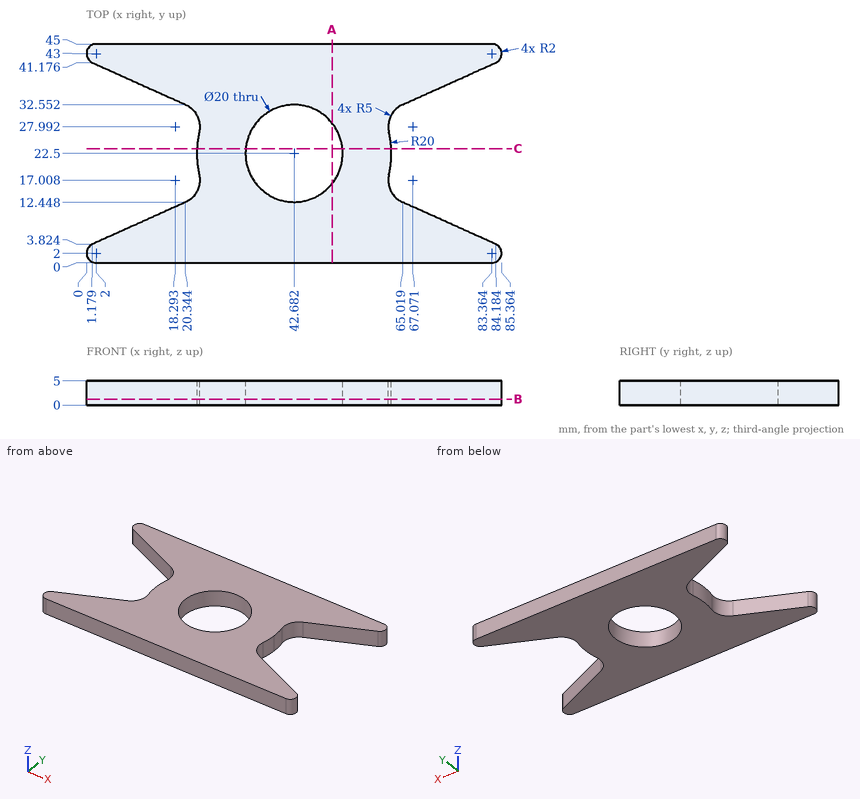
Design review of the part shown in the three views and the two pictorial views. Dimensions are in mm from the part's minimum x, y and z. Round coordinates to 2 decimals unless told otherwise and drop trailing zeros. Loops run counter-clockwise (first coordinate to the right, second up) from the corner with the lowest first, then second, coordinate; pieces in that order, holes last. Notation, with made-up numbers: (-2.75, 40) - (3.25, 40) arc R5 ccw to (3.25, 46) - close; hole circle Ø10 at (62.5, 20.5). An arc over 180 degrees is marked (long way). Write each question's results on one line, items separated by ' | '. Start each with the question number.
Q1. Insertion check: P1, Ø1.5, axis at y = 28, z = 1.5, coming from the -X side (1 decimal); P2, Ø1.5, axis at y = 27, z = 3, coming from the +X side. Each pin has a flat end and moves straight along its axis. Give the tip position at first contact, or say it passes through.
Q2. Wall thickness on line 1 along Y through (x, z) = (71, 4.55); line 2 along Y through (x, z) = (12.5, 2.15); line 3 along X through (y, z) = (29, 1.4) (1 decimal): over which ranges is each line inside the solid? List them lowest first. Write a range as [from, to].
Q3. Take a section at A-A on x = 50.5. Give the boundary of the cut face in (y, z) (1 decimal), plus the area to 3 significant figures.
Q4. Take a section at C-C on y = 23.5. Give the boundary of the cut face in (x, z).
Q5. Take a section at B-B on z = 1.25. Give the boundary of the cut face in (x, y) (1 decimal), plus the area to 3 significant figures.
Data:
1) P1: stops at x = 23.2 | P2: stops at x = 62.33
2) line 1: y = [0, 9.76], [35.24, 45] | line 2: y = [0, 8.92], [36.08, 45] | line 3: x = [23.2, 35.1], [50.3, 62.2]
3) outline: (0, 0) - (16.3, 0) - (16.3, 5) - (0, 5) - close; (28.7, 0) - (45, 0) - (45, 5) - (28.7, 5) - close | area: 163 mm²
4) outline: (22.71, 0) - (32.73, 0) - (32.73, 5) - (22.71, 5) - close; (52.63, 0) - (62.66, 0) - (62.66, 5) - (52.63, 5) - close
5) outline: (1.2, 3.8) arc R2 ccw to (2, 0) - (83.4, 0) arc R2 ccw to (84.2, 3.8) - (65, 12.4) arc R5 cw to (62.2, 18.1) arc R20 ccw to (62.7, 22.5) arc R20 ccw to (62.2, 26.9) arc R5 cw to (65, 32.6) - (84.2, 41.2) arc R2 ccw to (83.4, 45) - (2, 45) arc R2 ccw to (1.2, 41.2) - (20.3, 32.6) arc R5 cw to (23.2, 26.9) arc R20 ccw to (23.2, 18.1) arc R5 cw to (20.3, 12.4) - close; hole circle Ø20 at (42.7, 22.5) | area: 2,240 mm²
